Can you work these out from the model? Positions are in its coordinate system, mm. A direction names the side the tool comes from. Round coordinates to 2 decimals unless told otherwise and drop trailing zeros. Order: outer loops, then holes, each group sorted by start corner. A loop starts at its lowest first (then second) coordinate and runs counter-clockwise, first axis right, second up. Notation, with made-up numbers: (66, 71) - (74, 71) arc R16 cw to (74, 98) - close; hole circle Ø5 at (26.25, 5.5). An arc over 180 degrees is marked (long way). Write item = value, one per line.
from build123d import *

# Parameters (mm, degrees)
SKETCH1_R           = 75.565
SKETCH1_R_2         = 1.6
BOSS_EXTRUDE1_DEPTH = 6.35


with BuildPart() as part:
    # Sketch1 → Boss-Extrude1 (new body)
    with BuildSketch(Plane.XY):
        Circle(SKETCH1_R)
        with Locations((-51.308, 0)):
            Circle(SKETCH1_R_2, mode=Mode.SUBTRACT)
        with Locations(Location((51.308, 0, 0), (0, 0, 180))):
            Circle(SKETCH1_R_2, mode=Mode.SUBTRACT)
        with Locations((49.032198421, 49.032198421)):
            Circle(SKETCH1_R_2, mode=Mode.SUBTRACT)
        with Locations((49.032198421, -49.032198421)):
            Circle(SKETCH1_R_2, mode=Mode.SUBTRACT)
        with Locations((-49.032198421, -49.032198421)):
            Circle(SKETCH1_R_2, mode=Mode.SUBTRACT)
        with Locations((-49.032198421, 49.032198421)):
            Circle(SKETCH1_R_2, mode=Mode.SUBTRACT)
        with BuildLine():
            Line((-53.430637279, 12.065), (53.430637279, 12.065))
            ThreePointArc((53.430637279, 12.065), (58.600806141, 14.728286839), (59.434079669, 20.484101124))
            ThreePointArc((59.434079669, 20.484101124), (0, 62.865), (-59.434079669, 20.484101124))
            ThreePointArc((-59.434079669, 20.484101124), (-58.600806141, 14.728286839), (-53.430637279, 12.065))
        make_face(mode=Mode.SUBTRACT)
        with BuildLine():
            Line((-53.430637279, -12.065), (53.430637279, -12.065))
            ThreePointArc((53.430637279, -12.065), (58.600806141, -14.728286839), (59.434079669, -20.484101124))
            ThreePointArc((59.434079669, -20.484101124), (0, -62.865), (-59.434079669, -20.484101124))
            ThreePointArc((-59.434079669, -20.484101124), (-58.600806141, -14.728286839), (-53.430637279, -12.065))
        make_face(mode=Mode.SUBTRACT)
        with BuildLine():
            Line((-38.1, -3.556), (38.1, -3.556))
            ThreePointArc((38.1, -3.556), (39.896051224, -2.812051224), (40.64, -1.016))
            Line((40.64, -1.016), (40.64, 1.016))
            ThreePointArc((40.64, 1.016), (39.896051224, 2.812051224), (38.1, 3.556))
            Line((38.1, 3.556), (-38.1, 3.556))
            ThreePointArc((-38.1, 3.556), (-39.896051224, 2.812051224), (-40.64, 1.016))
            Line((-40.64, 1.016), (-40.64, -1.016))
            ThreePointArc((-40.64, -1.016), (-39.896051224, -2.812051224), (-38.1, -3.556))
        make_face(mode=Mode.SUBTRACT)
    extrude(amount=-BOSS_EXTRUDE1_DEPTH)


solid = part.part
(1) If we section it at D-D (x = 4): Write out the boundary of the cut face in (y, z) (3 decimals), plus the area to 3 significant figures.
Computed:
outline = (-75.459, -6.35) - (-62.738, -6.35) - (-62.738, 0) - (-75.459, 0) - close; (-12.065, -6.35) - (-3.556, -6.35) - (-3.556, 0) - (-12.065, 0) - close; (3.556, -6.35) - (12.065, -6.35) - (12.065, 0) - (3.556, 0) - close; (62.738, -6.35) - (75.459, -6.35) - (75.459, 0) - (62.738, 0) - close
area = 270 mm^2
(2) If we section it at A-A (x = -12): Write out the boundary of the cut face in (y, z) (3 decimals), plus the area to 3 significant figures.
Computed:
outline = (-74.606, -6.35) - (-61.709, -6.35) - (-61.709, 0) - (-74.606, 0) - close; (-12.065, -6.35) - (-3.556, -6.35) - (-3.556, 0) - (-12.065, 0) - close; (3.556, -6.35) - (12.065, -6.35) - (12.065, 0) - (3.556, 0) - close; (61.709, -6.35) - (74.606, -6.35) - (74.606, 0) - (61.709, 0) - close
area = 272 mm^2
(3) Thinking about a two-plate mould opening in X: for faces 3 (the face through (58.55, -14.66, -3.13)), 4 (the face through (-6, -5, 0)), 5 (the face through (-1, 12.065, -3)), 6 (the face through (72.076, 22.698, -3.131)), which applies, +X half, -X half, draft (parallel to the pull), parting line (faces both ways), or undercut?
Computed:
face_3 = undercut
face_4 = draft
face_5 = undercut
face_6 = parting line
(4) Will these pins go through, and if not, where does the flat tip stop? P1, Ø2, axis at y = -9.5, z = -3, coming from the -X side; P2, Ø3, axis at x = -5, z = -5.5, coming from the +Y side; P3, Ø2.5, axis at x = -49.03, y = -49.03, coming from the +Z side; P4, Ø3, axis at x = 34, z = -1.5, coming from the +Y side.
Computed:
P1 = -75.09
P2 = 75.48
P3 = through
P4 = 68.22
(5) On a 3-axis mill with a long thin cutter (end or side, diameter ignored), from which of +Z, -Z, +X, -X, +Y, -Y can I reach the whole of each face in a straight line? I mean faces 1 (the face through (-6, -5, -6.35)), 2 (the face through (1.09, 62.856, -3.131)). Say none if no direction works.
Computed:
face_1 = -Z, +X, -X, +Y, -Y
face_2 = +Z, -Z
(6) If I drill on line 1 (Y direction, x = -2, z = -5) (3 decimals); line 2 (Y direction, x = 55, z = -5.5); line 3 (Y direction, x = 44.5, z = -1) (3 decimals), over which ranges is the centre line in solid material (lowest first)? Write a range as from..to.
Computed:
line_1 = -75.539..-62.833, -12.065..-3.556, 3.556..12.065, 62.833..75.539
line_2 = -51.82..-30.45, -12.26..12.26, 30.45..51.82
line_3 = -61.072..-44.404, -12.065..12.065, 44.404..61.072
(7) If we section it at B-B (z = -3.5): State how many separate pieces and enclosed holes the cut face has, plus the area to 3 significant figures.
Computed:
separate_pieces = 1
enclosed_holes = 9
area = 7,980 mm^2
